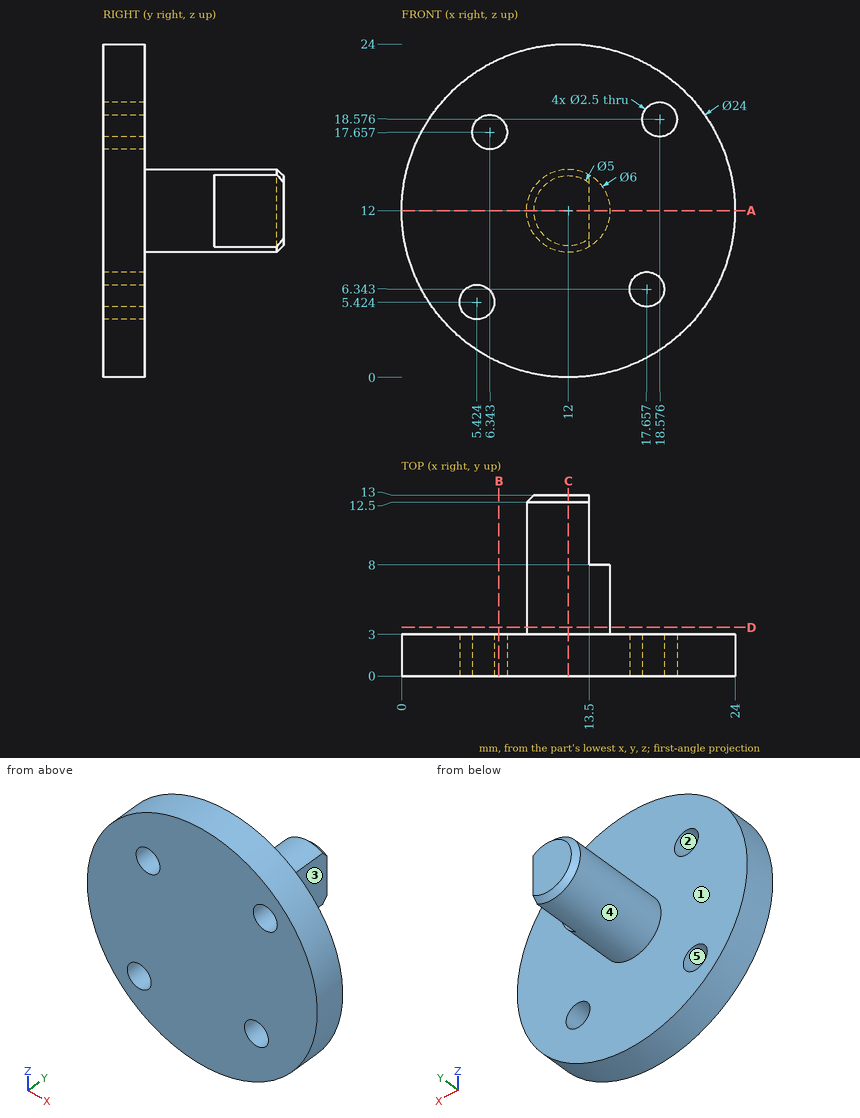
Verification items for this drawing (mm, ordinates from the low corner). A direction names the side the tool comes from. Round coordinates to 2 decimals unless told otherwise and drop trailing zeros. Write each loop counter-clockwise with the first axis right and the second up, starting at its lowest first coordinate (ties: lowest second). Pieces come first, ordered by that corner, then holes. Notation, with made-up numbers: (14, -16) - (19, -16) arc R16 cw to (19, -6) - close; hole circle Ø10 at (29.5, 7). An arc over 180 degrees is marked (long way). Answer as a JSON object with one key per item and string values. Group by question number.
Q1. Tool access check on the marked faces 1 and 2. Record the directions out of +Z, -Z, +X, -X, +Y, -Y that give a thin tool (end or side, any length) a straight path to the whole face; none if there is none.
Q2. Go/stop test with flat-tipped pins: pin 1 Ø10 at (x, z) = (7, 4) entering from +Y; pin 2 Ø10 at (x, z) = (16, 16.5) entering from -Y; pin 3 Ø1 at (y, z) = (5, 9.5) entering from -X; pin 4 Ø2 at (y, z) = (1.5, 10) entering from +X. Record where each tip stops, or that it passes through.
Q3. Section check B-B, the plane x = 7. Enter the section's corners in (y, z), plus the area to 3 significant figures.
Q4. Section check D-D, the plane y = 3.5. Enter the section's corners in (x, z), plus the area to 3 significant figures.
Q5. Section check A-A, the plane z = 12. Enter the section's corners in (x, y).
Q6. Mould release check, pull along Z, two halves, no side actions. Record for the marked faces 3, 4 and 5: released by +Z, released by -Z, zero draft, split by the parting line, or undercut.
Q7. Thickness scan on line 1 (Y direction, x = 19, z = 3); line 2 (Z direction, x = 10.25, y = 1); line 3 (X direction, y = 8.25, z = 13.75). Record the ranges inside material, lowest first.
Q8. Section check C-C, the plane x = 12. Enter the section's corners in (y, z).
Found:
{
 "1": {"face 1": "+Y", "face 2": "+Y, -Y"},
 "2": {"pin 1": "stops at y = 3", "pin 2": "stops at y = 0", "pin 3": "stops at x = 9.76", "pin 4": "stops at x = 23.96"},
 "3": {"outline": "(0, 1.09) - (3, 1.09) - (3, 16.59) - (0, 16.59) - close; (0, 18.72) - (3, 18.72) - (3, 22.91) - (0, 22.91) - close", "area": "59.1 mm^2"},
 "4": {"outline": "circle Ø6 at (12, 12)", "area": "28.3 mm^2"},
 "5": {"outline": "(0, 0) - (24, 0) - (24, 3) - (15, 3) - (15, 8) - (13.5, 8) - (13.5, 13) - (9.5, 13) - (9, 12.5) - (9, 3) - (0, 3) - close"},
 "6": {"face 3": "zero draft", "face 4": "split by the parting line", "face 5": "undercut"},
 "7": {"line 1": "y = 0 to 3", "line 2": "z = 0.13 to 23.87", "line 3": "x = 9.56 to 13.5"},
 "8": {"outline": "(0, 0) - (3, 0) - (3, 9) - (12.5, 9) - (13, 9.5) - (13, 14.5) - (12.5, 15) - (3, 15) - (3, 24) - (0, 24) - close"}
}
